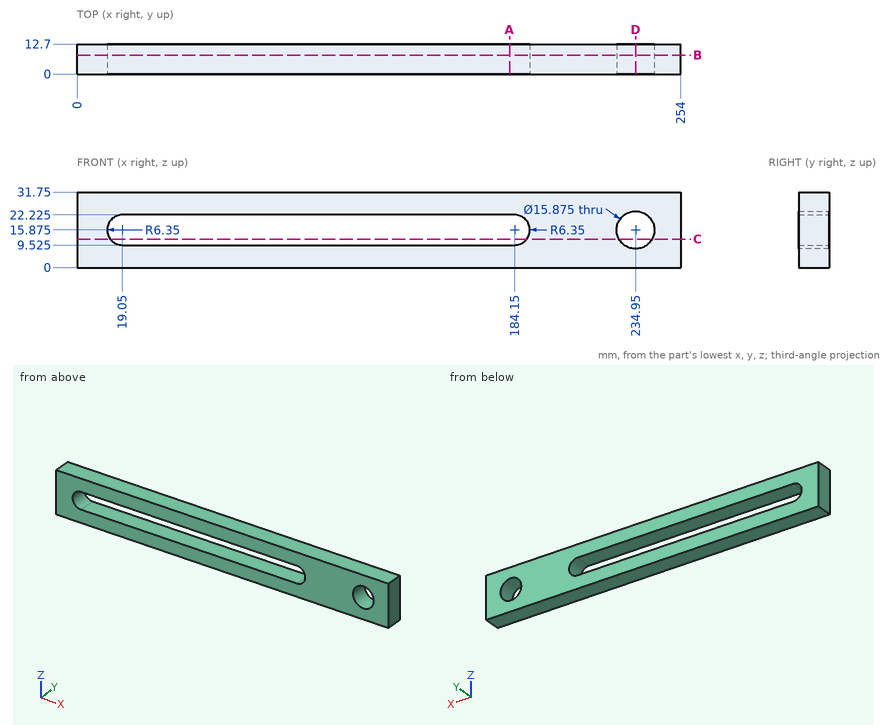
For this review, use the dimensioned drawing (mm, ordinates from the lowest corner) and the shaded views. Coordinates: 2 decimals unless noted, no trailing zeros. Write each loop counter-clockwise with the first axis right and the second up, starting at its lowest first coordinate (ties: lowest second). Pieces come first, ordered by that corner, then holes. Notation, with made-up numbers: (-26, 65) - (31, 65) arc R37 ccw to (31, 104) - close; hole circle Ø7 at (58, 15.25). An arc over 180 degrees is marked (long way). One line per item, written item: value.
1) Add section B-B (y = 8). Give the number of separate pieces and of enclosed holes in the cut face, plus the area to 3 significant figures.
Answer sheet:
separate pieces: 1
enclosed holes: 2
area: 5,640 mm2
2) To check wall thickness, follow probe 1 along X at (y, z) = (3.5, 15.5); probe 2 along Z at (x, y) = (101, 0.75) (3 decimals); probe 3 along X at (y, z) = (1.5, 14.5). State the ranges of each line that lie inside material, in increasing order.
Answer sheet:
probe 1: x = 0 to 12.71, 190.49 to 227.02, 242.88 to 254
probe 2: z = 0 to 9.525, 22.225 to 31.75
probe 3: x = 0 to 12.85, 190.35 to 227.13, 242.77 to 254
3) Add section D-D (x = 234.95). State the section outline as (y, z) points.
Answer sheet:
outline: (0, 0) - (12.7, 0) - (12.7, 7.94) - (0, 7.94) - close; (0, 23.81) - (12.7, 23.81) - (12.7, 31.75) - (0, 31.75) - close
4) Add section C-C (z = 12). State the section outline as (x, y) points, plus the area to 3 significant figures.
Answer sheet:
outline: (0, 0) - (14.02, 0) - (14.02, 12.7) - (0, 12.7) - close; (189.18, 0) - (228.02, 0) - (228.02, 12.7) - (189.18, 12.7) - close; (241.88, 0) - (254, 0) - (254, 12.7) - (241.88, 12.7) - close
area: 825 mm2
5) Add section A-A (x = 182). State the section outline as (y, z) points (3 decimals).
Answer sheet:
outline: (0, 0) - (12.7, 0) - (12.7, 9.525) - (0, 9.525) - close; (0, 22.225) - (12.7, 22.225) - (12.7, 31.75) - (0, 31.75) - close
